Here's how the part is built. I have some questions about the finished solid (model axes, mm). Give positions to 0.01 mm unless a question says otherwise; leave off trailing zeros. Loops run counter-clockwise (first coordinate to the right, second up) from the corner with the lowest first, then second, coordinate; pieces in that order, holes last.
Q1. Suppose I cut it at A-A (x = 12.7). List the corners of the cut face in (y, z) for me (3 decimals), and give its area (3 significant figures).
Q2. I need wall thicknesses on probe 1 along X at (y, z) = (46.5, 0.8); probe 2 along X at (y, z) = (5, 0.35); probe 3 along X at (y, z) = (3.5, 0.4). Which ranges of each line are inside material? Lowest first, please.
Q3. Suppose I cut it at B-B (x = -6). List the corners of the cut face in (y, z) for me.
Q4. Suppose I cut it at C-C (y = 53). List the corners of the cut face in (x, z) for me.
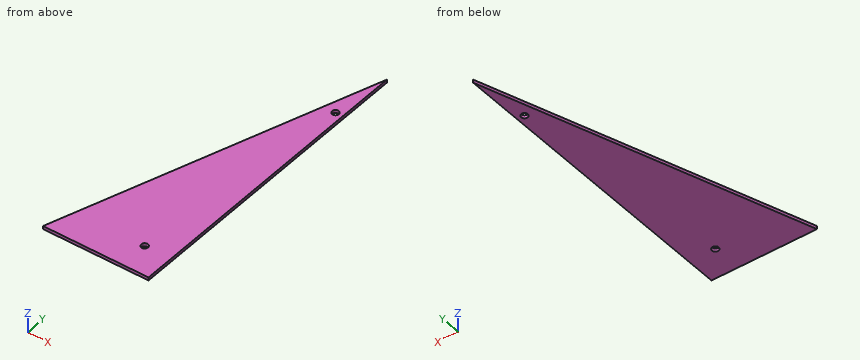
```python
from build123d import *

# Parameters (mm, degrees)
F1_DEPTH = 1.524
F2_R     = 1.6129
F3_DEPTH = 25.4
F4_DEPTH = 39.37


with BuildPart() as f1:
    # F0 (on Top) → F1 (new body)
    with BuildSketch(Plane.XY):
        Polygon((-25.4, -74.93), (25.4, -74.93), (25.4, 74.93), align=None)
    extrude(amount=F1_DEPTH)

    # F2 (on face) → F3 (cut)
    with BuildSketch(Plane.XY.offset(1.524)):
        with Locations((21.858884, 47.176842)):
            Circle(F2_R)
        with Locations((12.7, -60.773158)):
            Circle(F2_R)
    extrude(amount=-F3_DEPTH, mode=Mode.SUBTRACT)

    # F2 (on face) → F4 (cut)
    with BuildSketch(Plane.XY.offset(1.524)):
        with Locations((21.858884, 47.176842)):
            Circle(F2_R)
        with Locations((12.7, -60.773158)):
            Circle(F2_R)
    extrude(amount=F4_DEPTH, mode=Mode.SUBTRACT)


solid = f1.part
```
Solutions:
1. outline: (-74.93, 0) - (-62.386, 0) - (-62.386, 1.524) - (-74.93, 1.524) - close; (-59.16, 0) - (37.465, 0) - (37.465, 1.524) - (-59.16, 1.524) - close
1. area: 166 mm2
2. probe 1: x = 15.76 to 20.39, 23.32 to 25.4
2. probe 2: x = 1.69 to 25.4
2. probe 3: x = 1.19 to 25.4
3. outline: (-74.93, 0) - (-17.7, 0) - (-17.7, 1.52) - (-74.93, 1.52) - close
4. outline: (17.97, 0) - (25.4, 0) - (25.4, 1.52) - (17.97, 1.52) - close
